Can you work these out from the model? Positions are in its coordinate system, mm. A direction names the side the tool comes from. Round coordinates to 2 decimals unless told otherwise and drop trailing zeros. Order: outer loops, then holes, each group sorted by start corner. A loop starts at its lowest first (then second) coordinate and runs counter-clockwise, first axis right, second up. Notation, with made-up numbers: (71, 16) -> (92, 16) arc R23 cw to (92, 46) -> close; hole circle Ø11 at (10, 65.25). An arc over 180 degrees is marked (long way). Use a Markdown table: item, result. Add a question column.
Q1. I'm going to push flat-ended pins straight in: pin 1 Ø1.5 at (y, z) = (25.5, 15.5) entering from +X; pin 2 Ø5 at (x, z) = (15, 10) entering from -Y; pin 3 Ø3.5 at (y, z) = (8, 7) entering from +X. Where does each tip first touch, or does it pass through?
Q2. If we section it at A-A on y = 38.5: List the corners of the cut face in (x, z) for me.
Q3. If we section it at D-D on z = 7.25: List the corners of the cut face in (x, y) for me, plus the area to 3 significant figures.
Q4. If we section it at B-B on x = 27.55: List the corners of the cut face in (y, z) for me, plus the area to 4 significant figures.
Q5. If we section it at C-C on x = 13: List the corners of the cut face in (y, z) for me, plus the area to 3 significant figures.
Q6. We'd pull the mould along X, two halves only. Please class faces 5 (the face through (32.4, 14, 6)), 6 (the face through (35.285, 13.951, 2.826)), 7 (the face through (36.4, 21, 3)): +X half, -X half, draft (parallel to the pull), parting line (faces both ways), or undercut.
Q7. I need wall thicknesses on line 1 along Y through (x, z) = (24, 4.25); line 2 along Z through (x, y) = (34.5, 15); line 3 along Y through (x, z) = (2.2, 5.85). Which ranges of each line are inside material? Lowest first, please. Write a range as [from, to].
Q8. For faces 1 (the face through (3.7, 19.6, 11.7)), 2 (the face through (31.83, 23.4, 5.93)), 3 (the face through (6.2, 34, 2)), 4 (the face through (11, 27, 6)), which set-ups out of +Z, -Z, +X, -X, +Y, -Y let a thin tool reach every point of the face, with its end or its side?
```python
from build123d import *

# Parameters (mm, degrees)
SKETCH_1_R          = 1
EXTRUDE_1_DEPTH     = 4.6
EXTRUDE_2_DEPTH     = 11.7
SKETCH_1_4_W        = 12
SKETCH_1_4_H        = 3
EXTRUDE_3_DEPTH     = 11.7
SKETCH_2_R          = 3.65
CUT_EXTRUDE_1_DEPTH = 24.5
CUT_EXTRUDE_2_DEPTH = 2.2
FILLET_2_R          = 5.85
FILLET_3_R          = 5.85
FILLET_4_R          = 5.85
FILLET_1_R          = 5.85
FILLET_5_R          = 2
FILLET_6_R          = 2
FILLET_8_R          = 2
SKETCH_3_R          = 2.95
CUT_EXTRUDE_3_DEPTH = 10
SKETCH_1_6_R        = 0.85
EXTRUDE_5_DEPTH     = 17.5
FILLET_9_R          = 2
CUT_EXTRUDE_START   = -2.2
CUT_EXTRUDE_4_DEPTH = 2.2
CUT_EXTRUDE_START_2 = -10.2
SKETCH_4_3_R        = 3.65
SKETCH_4_3_R_2      = 2.95
CUT_EXTRUDE_5_DEPTH = 10.2
EXTRUDE_6_DEPTH     = 2.2
SKETCH_2_5_R        = 3.65
EXTRUDE_7_DEPTH     = 4
SKETCH_5_R          = 2.95
CUT_EXTRUDE_6_DEPTH = 8.2


with BuildPart() as part:
    # 草图1 → 凸台-拉伸1 (new body)
    with BuildSketch(Plane.XY):
        Polygon((0, 44.5), (0, 27), (6.2, 27), (6.2, 28), (6.2, 41), (30.2, 41), (30.2, 28), (29.9, 28), (29.9, 27), (30.2, 27), (35, 27), (36.4, 27), (36.4, 44.5), align=None)
        with Locations((4.2, 34.5)):
            Circle(SKETCH_1_R, mode=Mode.SUBTRACT)
        with Locations((32.2, 34.5)):
            Circle(SKETCH_1_R, mode=Mode.SUBTRACT)
    extrude(amount=EXTRUDE_1_DEPTH)

    # 草图1<3> → 凸台-拉伸2 (add)
    with BuildSketch(Plane.XY):
        Polygon((0, 27), (0, 0), (4, 0), (4, 24), (6.2, 24), (6.2, 27), align=None)
        Polygon((36.4, 0), (36.4, 27), (30.2, 27), (30.2, 24), (32.4, 24), (32.4, 0), align=None)
    extrude(amount=EXTRUDE_2_DEPTH)

    # 草图1<4> → 凸台-拉伸3 (add)
    with BuildSketch(Plane.XY):
        with Locations((12.2, 25.5)):
            Rectangle(SKETCH_1_4_W, SKETCH_1_4_H)
    extrude(amount=EXTRUDE_3_DEPTH)

    # 草图2 → 切除-拉伸1 (cut)
    with BuildSketch(Plane.ZY):
        with Locations((5.85, 5.85)):
            Circle(SKETCH_2_R)
    extrude(amount=-CUT_EXTRUDE_1_DEPTH, mode=Mode.SUBTRACT)

    # 草图2<3> → 切除-拉伸2 (cut)
    with BuildSketch(Plane.ZY):
        with BuildLine():
            Line((9.488773874, 6.136050157), (8.242618438, 21.988087774))
            ThreePointArc((8.242618438, 21.988087774), (5.85, 24.2), (3.457381562, 21.988087774))
            Line((3.457381562, 21.988087774), (2.211226126, 6.136050157))
            ThreePointArc((2.211226126, 6.136050157), (5.85, 9.5), (9.488773874, 6.136050157))
        make_face()
    extrude(amount=-CUT_EXTRUDE_2_DEPTH, mode=Mode.SUBTRACT)

    # 圆角2
    fillet_2_edges = [part.edges().sort_by_distance(p)[0] for p in [
        (2, 0, 0),
    ]]
    fillet(fillet_2_edges, radius=FILLET_2_R)

    # 圆角3
    fillet_3_edges = [part.edges().sort_by_distance(p)[0] for p in [
        (34.4, 0, 0),
    ]]
    fillet(fillet_3_edges, radius=FILLET_3_R)

    # 圆角4
    fillet_4_edges = [part.edges().sort_by_distance(p)[0] for p in [
        (34.4, 0, 11.7),
    ]]
    fillet(fillet_4_edges, radius=FILLET_4_R - 0.0001)  # a hair under: the kernel refuses the full size

    # 圆角1
    fillet_1_edges = [part.edges().sort_by_distance(p)[0] for p in [
        (2, 0, 11.7),
    ]]
    fillet(fillet_1_edges, radius=FILLET_1_R - 0.0001)  # a hair under: the kernel refuses the full size

    # 圆角5
    fillet_5_edges = [part.edges().sort_by_distance(p)[0] for p in [
        (0, 44.5, 2.3),
    ]]
    fillet(fillet_5_edges, radius=FILLET_5_R)

    # 圆角6
    fillet_6_edges = [part.edges().sort_by_distance(p)[0] for p in [
        (36.4, 44.5, 2.3),
    ]]
    fillet(fillet_6_edges, radius=FILLET_6_R)

    # 圆角8
    fillet_8_edges = [part.edges().sort_by_distance(p)[0] for p in [
        (4, 24, 5.85),
    ]]
    fillet(fillet_8_edges, radius=FILLET_8_R)

    # 草图3 → 切除-拉伸3 (cut)
    with BuildSketch(Plane(origin=(36.4, 0, 0), x_dir=(0, 0, -1), z_dir=(1, 0, 0))):
        with Locations(Location((-5.85, 5.85, 0), (0, 0, 90))):
            Circle(SKETCH_3_R)
    extrude(amount=-CUT_EXTRUDE_3_DEPTH, mode=Mode.SUBTRACT)

    # 草图1<6> → 凸台-拉伸5 (add)
    with BuildSketch(Plane.XY):
        Polygon((18.2, 28), (18.2, 27), (18.2, 24), (30.2, 24), (30.2, 27), (29.9, 27), (29.9, 28), align=None)
        with Locations((20.55, 26)):
            Circle(SKETCH_1_6_R, mode=Mode.SUBTRACT)
        with Locations((27.55, 26)):
            Circle(SKETCH_1_6_R, mode=Mode.SUBTRACT)
    extrude(amount=EXTRUDE_5_DEPTH)

    # 圆角9
    fillet_9_edges = [part.edges().sort_by_distance(p)[0] for p in [
        (32.4, 24, 5.85),
    ]]
    fillet(fillet_9_edges, radius=FILLET_9_R)

    # 草图4 → 切除-拉伸4 (cut)
    with BuildSketch(Plane(origin=(36.4, 0, 0), x_dir=(0, 0, -1), z_dir=(1, 0, 0)).offset(CUT_EXTRUDE_START)):
        with BuildLine():
            ThreePointArc((-3.457381562, 21.988087774), (-5.85, 24.2), (-8.242618438, 21.988087774))
            Line((-8.242618438, 21.988087774), (-9.488773874, 6.136050157))
            ThreePointArc((-9.488773874, 6.136050157), (-5.85, 9.5), (-2.211226126, 6.136050157))
            Line((-2.211226126, 6.136050157), (-3.457381562, 21.988087774))
        make_face()
    extrude(amount=CUT_EXTRUDE_4_DEPTH, mode=Mode.SUBTRACT)

    # 草图4<3> → 切除-拉伸5 (cut)
    with BuildSketch(Plane(origin=(36.4, 0, 0), x_dir=(0, 0, -1), z_dir=(1, 0, 0)).offset(CUT_EXTRUDE_START_2)):
        with Locations(Location((-5.85, 5.85, 0), (0, 0, 175.505125981))):
            Circle(SKETCH_4_3_R)
        with Locations((-5.85, 5.85)):
            Circle(SKETCH_4_3_R_2, mode=Mode.SUBTRACT)
    extrude(amount=CUT_EXTRUDE_5_DEPTH, mode=Mode.SUBTRACT)

    # 草图2<4> → 凸台-拉伸6 (add)
    with BuildSketch(Plane.ZY):
        with BuildLine():
            Line((9.488773874, 6.136050157), (8.242618438, 21.988087774))
            ThreePointArc((8.242618438, 21.988087774), (5.85, 24.2), (3.457381562, 21.988087774))
            Line((3.457381562, 21.988087774), (2.211226126, 6.136050157))
            ThreePointArc((2.211226126, 6.136050157), (5.85, 9.5), (9.488773874, 6.136050157))
        make_face()
    extrude(amount=-EXTRUDE_6_DEPTH)

    # 草图2<5> → 凸台-拉伸7 (add)
    with BuildSketch(Plane.ZY):
        with Locations(Location((5.85, 5.85, 0), (0, 0, 4.494874019))):
            Circle(SKETCH_2_5_R)
    extrude(amount=-EXTRUDE_7_DEPTH)

    # 草图5 → 切除-拉伸6 (cut)
    with BuildSketch(Plane.ZY):
        with Locations((5.85, 5.85)):
            Circle(SKETCH_5_R)
    extrude(amount=-CUT_EXTRUDE_6_DEPTH, mode=Mode.SUBTRACT)


solid = part.part
```
Answer below:
| question | item | result |
|---|---|---|
| 1 | pin 1 | x = 30.2 |
| 1 | pin 2 | y = 24 |
| 1 | pin 3 | x = 34.2 |
| 2 | outline | (0, 0) -> (6.2, 0) -> (6.2, 4.6) -> (0, 4.6) -> close; (30.2, 0) -> (36.4, 0) -> (36.4, 4.6) -> (30.2, 4.6) -> close |
| 3 | outline | (0, 0.17) -> (4, 0.17) -> (4, 3.25) -> (0, 3.25) -> close; (0, 8.45) -> (4, 8.45) -> (4, 22) arc R2 cw to (6, 24) -> (30.4, 24) arc R2 cw to (32.4, 22) -> (32.4, 9.22) -> (34.2, 9.22) -> (34.2, 23.75) -> (36.4, 23.75) -> (36.4, 27) -> (29.9, 27) -> (29.9, 28) -> (18.2, 28) -> (18.2, 27) -> (0, 27) -> close; (32.4, 0.17) -> (36.4, 0.17) -> (36.4, 2.48) -> (32.4, 2.48) -> close; hole circle Ø1.7 at (20.55, 26); hole circle Ø1.7 at (27.55, 26) |
| 3 | area | 229 mm² |
| 4 | outline | (24, 0) -> (25.15, 0) -> (25.15, 17.5) -> (24, 17.5) -> close; (26.85, 0) -> (28, 0) -> (28, 17.5) -> (26.85, 17.5) -> close; (41, 0) -> (44.5, 0) -> (44.5, 4.6) -> (41, 4.6) -> close |
| 4 | area | 56.35 mm² |
| 5 | outline | (24, 0) -> (27, 0) -> (27, 11.7) -> (24, 11.7) -> close; (41, 0) -> (44.5, 0) -> (44.5, 4.6) -> (41, 4.6) -> close |
| 5 | area | 51.2 mm² |
| 6 | face 5 | undercut |
| 6 | face 6 | draft |
| 6 | face 7 | +X half |
| 7 | line 1 | [24, 28], [41, 44.5] |
| 7 | line 2 | [0, 2.91], [8.79, 11.7] |
| 7 | line 3 | [0, 2.9], [8.8, 27] |
| 8 | face 1 | +Z, -X, +Y, -Y |
| 8 | face 2 | +Z, -Z, -Y |
| 8 | face 3 | +Z, -Z |
| 8 | face 4 | +Z |
